Part print with two shaded views. Sizes in mm from the minimum x, y, z corner. Round coordinates to 2 decimals unless told otherwise and drop trailing zeros. Write each loop counter-clockwise with the first axis right and the second up, starting at its lowest first coordinate (ties: lowest second). Pieces come first, ordered by that corner, then holes. Notation, with made-up numbers: (1, 9.25) -> (31, 9.25) arc R12 ccw to (31, 30.25) -> close; hole circle Ø1 at (14.25, -24.5). An arc over 180 degrees is marked (long way). Return JSON: item names as keys, results as strings. Group by question number.
(1) Drill centre line: L1, parallel to Z at x = 956, y = 218.5. Where is it in solid material? Low to high. Write a range as from..to.
(2) Saw through at B-B (y = 40). List the corners of the cut face in (x, z).
(3) Saw through at A-A (x = 40). List the corners of the cut face in (y, z).
(4) Saw through at D-D (y = 369.5). List the corners of the cut face in (x, z).
(5) Saw through at C-C (z = 727). List the corners of the cut face in (x, y).
(6) Drop a flat-ended pin along its axis: pin 1 Ø8 at (x, y) = (595, 320) entering from -Z. Give the stop position or say it passes through.
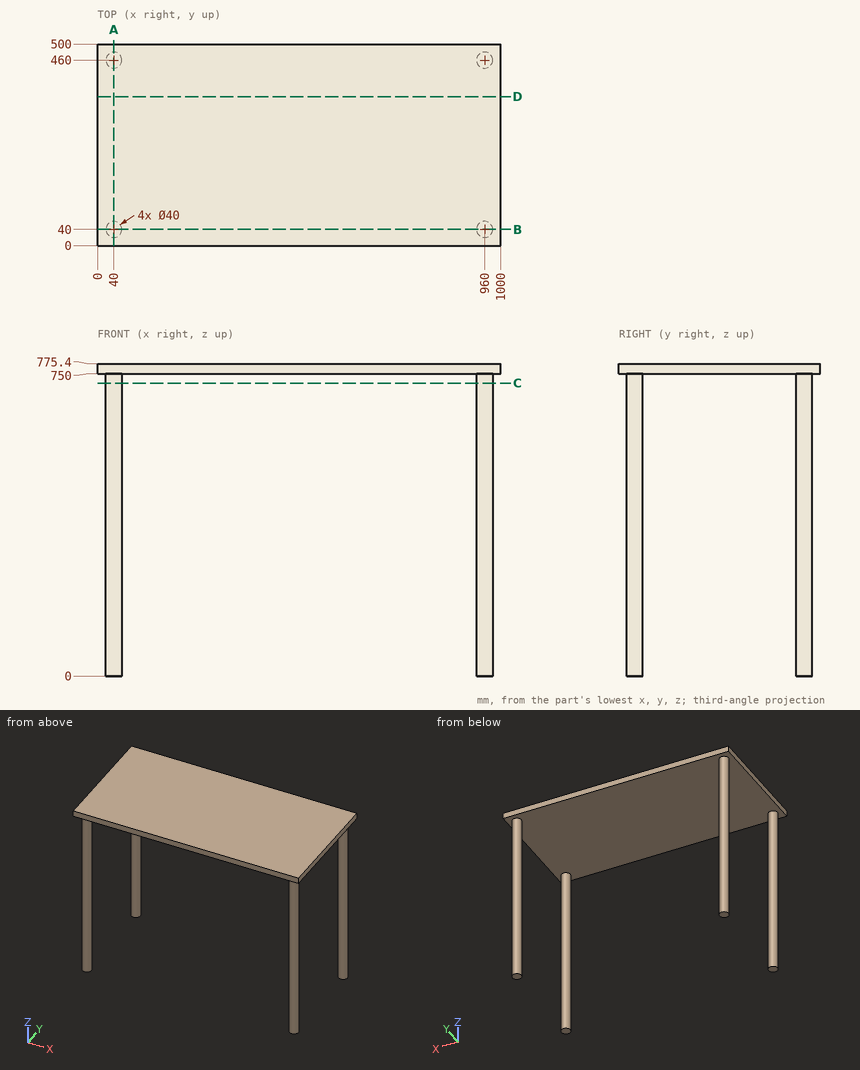
Computed values:
{
 "1": {"L1": "750..775.4"},
 "2": {"outline": "(0, 750) -> (20, 750) -> (20, 0) -> (60, 0) -> (60, 750) -> (940, 750) -> (940, 0) -> (980, 0) -> (980, 750) -> (1000, 750) -> (1000, 775.4) -> (0, 775.4) -> close"},
 "3": {"outline": "(0, 750) -> (20, 750) -> (20, 0) -> (60, 0) -> (60, 750) -> (440, 750) -> (440, 0) -> (480, 0) -> (480, 750) -> (500, 750) -> (500, 775.4) -> (0, 775.4) -> close"},
 "4": {"outline": "(0, 750) -> (1000, 750) -> (1000, 775.4) -> (0, 775.4) -> close"},
 "5": {"outline": "circle Ø40 at (40, 40); circle Ø40 at (40, 460); circle Ø40 at (960, 40); circle Ø40 at (960, 460)"},
 "6": {"pin 1": "z = 750"}
}
